```python
from build123d import *

# Parameters (mm, degrees)
F1_DEPTH = 3


# Not quite as in the source:
# - a feature names something its author has since deleted; it is built from what else it names


with BuildPart() as f1:
    # F0 (on Top) → F1 (new body)
    with BuildSketch(Plane.XY):
        with BuildLine():
            Line((8.3654914828, 7.7478343503), (8.3654914828, 25.7808157751))
            ThreePointArc((8.3654914828, 25.7808157751), (0.4767203504, 33.9966565171), (-7.631576467, 25.9973895632))
            Line((-7.631576467, 25.9973895632), (-8.6528857034, 7.4260866897))
            ThreePointArc((-8.6528857034, 7.4260866897), (-9.3855131516, 5.0826540918), (-11.1453419747, 3.3705145438))
            Line((-11.1453419747, 3.3705145438), (-26.7623619946, -5.6459761686))
            ThreePointArc((-26.7623619946, -5.6459761686), (-29.9331032244, -16.585772745), (-18.951386422, -19.6081302933))
            Line((-18.951386422, -19.6081302933), (-2.3575117339, -11.2069586004))
            ThreePointArc((-2.3575117339, -11.2069586004), (0.038274152, -10.6697162831), (2.400944907, -11.3377029763))
            Line((2.400944907, -11.3377029763), (18.0179649268, -20.3541936886))
            ThreePointArc((18.0179649268, -20.3541936886), (29.0774772891, -17.6302378543), (26.204057304, -6.6086133521))
            Line((26.204057304, -6.6086133521), (10.6314918524, 3.5615178285))
            ThreePointArc((10.6314918524, 3.5615178285), (8.9683334147, 5.3677081091), (8.3654914828, 7.7478343503))
        make_face()
        with BuildLine():
            ThreePointArc((-20.451386422, -12.679927063), (-25.3707248656, -13.3098488797), (-20.7688276181, -11.4607318089))
            ThreePointArc((-20.7688276181, -11.4607318089), (-20.5320479783, -12.0500052463), (-20.451386422, -12.679927063))
        make_face(mode=Mode.SUBTRACT)
        with BuildLine():
            ThreePointArc((24.704057304, -13.5368165824), (21.5399163779, -15.9469860432), (20.0569238399, -12.25626284))
            ThreePointArc((20.0569238399, -12.25626284), (22.8681982302, -11.1266471215), (24.704057304, -13.5368165824))
        make_face(mode=Mode.SUBTRACT)
        with BuildLine():
            ThreePointArc((-7.9164689421, -4.2812988086), (-7.6979940139, 4.6627125327), (0.127531223, 8.9990963873))
            ThreePointArc((0.127531223, 8.9990963873), (6.4088915191, 6.3187110629), (9, 0))
            ThreePointArc((9, 0), (8.6421794957, -2.5125153857), (7.5971703192, -4.8252464332))
            ThreePointArc((7.5971703192, -4.8252464332), (-0.315369081, -8.9944728774), (-7.9164689421, -4.2812988086))
        make_face(mode=Mode.SUBTRACT)
        with BuildLine():
            ThreePointArc((2.868423533, 25.9973895632), (2.1236210505, 24.217141919), (0.3329981933, 23.4976405667))
            ThreePointArc((0.3329981933, 23.4976405667), (-1.3867739845, 27.7776372074), (2.868423533, 25.9973895632))
        make_face(mode=Mode.SUBTRACT)
        with BuildLine():
            ThreePointArc((0.0354253397, 2.4997489965), (1.7802476442, 1.7551975175), (2.5, 0))
            ThreePointArc((2.5, 0), (2.3734655501, -0.7852778377), (2.0066709741, -1.4910639161))
            Line((2.0066709741, -1.4910639161), (7.5971703192, -4.8252464332))
            ThreePointArc((7.5971703192, -4.8252464332), (8.6421794957, -2.5125153857), (9, 0))
            ThreePointArc((9, 0), (6.4088915191, 6.3187110629), (0.127531223, 8.9990963873))
            Line((0.127531223, 8.9990963873), (0.0354253397, 2.4997489965))
        make_face()
        with BuildLine():
            ThreePointArc((-2.239906233, -1.1103243073), (-2.1149683962, 1.333007383), (0.0354253397, 2.4997489965))
            Line((0.0354253397, 2.4997489965), (0.127531223, 8.9990963873))
            ThreePointArc((0.127531223, 8.9990963873), (-7.6979940139, 4.6627125327), (-7.9164689421, -4.2812988086))
            Line((-7.9164689421, -4.2812988086), (-2.239906233, -1.1103243073))
        make_face()
        with BuildLine():
            Line((7.5971703192, -4.8252464332), (2.0066709741, -1.4910639161))
            ThreePointArc((2.0066709741, -1.4910639161), (-0.2232494881, -2.4900119811), (-2.239906233, -1.1103243073))
            Line((-2.239906233, -1.1103243073), (-7.9164689421, -4.2812988086))
            ThreePointArc((-7.9164689421, -4.2812988086), (-0.315369081, -8.9944728774), (7.5971703192, -4.8252464332))
        make_face()
    extrude(amount=F1_DEPTH)


solid = f1.part
```
The model under review builds one solid part; all positions refer to its coordinate system, in mm. A direction names the side the tool comes from. Round coordinates to 2 decimals unless told otherwise and drop trailing zeros. Loops run counter-clockwise (first coordinate to the right, second up) from the corner with the lowest first, then second, coordinate; pieces in that order, holes last. Notation, with made-up numbers: (80.5, 63.25) -> (118.5, 63.25) arc R8 cw to (118.5, 67.25) -> close; hole circle Ø4 at (78, 14.25). An arc over 180 degrees is marked (long way). Answer in a Markdown table with one row per item.
1) Consider section B-B, the plane y = 1. Write out the cut boundary in (x, z).
Taken from the geometry:
| item | result |
|---|---|
| outline | (-15.25, 0) -> (-2.29, 0) -> (-2.29, 3) -> (-15.25, 3) -> close; (2.29, 0) -> (14.55, 0) -> (14.55, 3) -> (2.29, 3) -> close |
2) Draft analysis for pull direction X (two halves, no side actions). For faces 4 (the flat face through (18.527, -1.595, 1.479)), 5 (the flat face through (-18.84, -1.07, 1.48)), 6 (the flat face through (-10.771, -15.466, 1.479)), state which applies: pulls with the +X half, pulls with the -X half, needs draft (parallel to the pull), parting line crosses it, or undercut.
Taken from the geometry:
| item | result |
|---|---|
| face 4 | pulls with the +X half |
| face 5 | pulls with the -X half |
| face 6 | undercut |
3) Consider section D-D, the plane y = 16. Write out the cut boundary in (x, z).
Taken from the geometry:
| item | result |
|---|---|
| outline | (-8.18, 0) -> (8.37, 0) -> (8.37, 3) -> (-8.18, 3) -> close |
4) Tool access review of faces 1 (the flat face through (8.365, 17, 1)), 2 (the flat face through (10.1, -15.783, 1.479)), 3 (the flat face through (-8.135, 16.842, 1.479)): name each direction out of +Z, -Z, +X, -X, +Y, -Y from which nothing blocks a thin tool from reaching the whole face with its end or side.
Taken from the geometry:
| item | result |
|---|---|
| face 1 | +Z, -Z, +X, +Y |
| face 2 | +Z, -Z, -Y |
| face 3 | +Z, -Z, -X, +Y |
5) Wall thickness on line 1 along X through (y, z) = (-13.5, 1.85); line 2 along X through (y, z) = (-15.5, 0.2); line 3 along X through (y, z) = (-10.5, 2.65): over which ranges is each line inside the solid? List them lowest first.
Taken from the geometry:
| item | result |
|---|---|
| line 1 | x = -30.91 to -25.31, -20.59 to -6.89, 6.15 to 19.7, 24.7 to 30.2 |
| line 2 | x = -30.44 to -10.84, 9.61 to 20.66, 23.75 to 29.96 |
| line 3 | x = -30.65 to -24.18, -21.73 to 29.61 |
6) Consider section A-A, the plane z = 1.75. Write out the cut boundary in (x, y).
Taken from the geometry:
| item | result |
|---|---|
| outline | (-26.76, -5.65) arc R8 ccw (long way) to (-18.95, -19.61) -> (-2.36, -11.21) arc R5 cw to (2.4, -11.34) -> (18.02, -20.35) arc R8 ccw (long way) to (26.2, -6.61) -> (10.63, 3.56) arc R5 cw to (8.37, 7.75) -> (8.37, 25.78) arc R8 ccw (long way) to (-7.63, 26) -> (-8.65, 7.43) arc R5 cw to (-11.15, 3.37) -> close; hole circle Ø5 at (-22.95, -12.68); hole circle Ø5 at (0, 0); hole circle Ø5 at (0.37, 26); hole circle Ø5 at (22.2, -13.54) |
7) Consider section C-C, the plane x = -5. Write out the cut boundary in (y, z), plus the area to 3 significant figures.
Taken from the geometry:
| item | result |
|---|---|
| outline | (-12.54, 0) -> (31.93, 0) -> (31.93, 3) -> (-12.54, 3) -> close |
| area | 133 mm² |
8) For pin 1 Ø4 at (x, y) = (0.37, 26) entering from -Z; pin 2 Ø1.5 at (y, z) = (15.5, 2) entering from +X, all flat-tipped, find the tip position at first contact; note any pin that passes through.
Taken from the geometry:
| item | result |
|---|---|
| pin 1 | passes through |
| pin 2 | stops at x = 8.37 |
